Check sheet for the modelled part. Datum: model origin and axes. Units: mm. Face numbers are marked on the shaded views. Give positions to 0.01 mm unless a question says otherwise; leave off trailing zeros. Order: outer loops, then holes, each group sorted by start corner. A loop starts at its lowest first (then second) coordinate and runs counter-clockwise, first axis right, second up.
Item 1: Sectioned sample at A-A on x = 76.2. Record the boundary of the cut face in (y, z) (1 decimal).
Item 2: Release check for a two-part mould opening along Y. For the marked faces 1, 2, 3 and 4 record: released by +Y, released by -Y, zero draft, split by the parting line, or undercut.
Item 3: Sectioned sample at C-C on y = 6.5. Count the separate pieces of the cut face and the enclosed holes in it, and give its area (3 significant figures).
Item 4: Gauge pin test, flat ends, axial feed: P1, Ø6.5, axis at x = 109.54, y = 7.94, coming from the +Z side; P2, Ø7.5, axis at x = 46.04, y = 7.94, coming from the -Z side. Record the tip position at first contact, or that the pin passes through.
Item 5: Sectioned sample at B-B on x = 63.5. Record the boundary of the cut face in (y, z) (3 decimals).
Item 6: Material ranges on line 1 along X through (y, z) = (4.5, 12.25) (3 decimals); line 2 along X through (y, z) = (10, 7) (3 decimals); line 3 along X through (y, z) = (8.5, 13) (3 decimals), recorded low to high.
from build123d import *

# Parameters (mm, degrees)
F0_W     = 117.475
F0_H     = 15.875
F1_DEPTH = 25.4
F2_R     = 3.96875
F2_R_2   = 3.175
F2_R_3   = 5.55625
F3_DEPTH = 25.401
F4_R     = 3.175
F4_R_2   = 2.38125
F5_DEPTH = 15.876
F6_SIZE  = 0.762


with BuildPart() as f1:
    # F0 (on Top) → F1 (new body)
    with BuildSketch(Plane.XY):
        with Locations((58.7375, 7.9375)):
            Rectangle(F0_W, F0_H)
    extrude(amount=F1_DEPTH)

    # F2 (on face) → F3 (cut, through all)
    with BuildSketch(Plane.XY.offset(25.4)):
        with Locations((7.9375, 7.9375)):
            Circle(F2_R)
        with Locations((46.0375, 7.9375)):
            Circle(F2_R_2)
        with Locations((63.5, 7.9375)):
            Circle(F2_R_3)
        with Locations((109.5375, 7.9375)):
            Circle(F2_R)
    extrude(amount=-F3_DEPTH, mode=Mode.SUBTRACT)

    # F4 (on face) → F5 (cut, through all)
    with BuildSketch(Plane.XZ):
        with Locations((76.2, 17.4625)):
            Circle(F4_R)
        with Locations((90.4875, 5.5626)):
            Circle(F4_R_2)
    extrude(amount=-F5_DEPTH, mode=Mode.SUBTRACT)

    # F6
    f6_edges = [f1.edges().sort_by_distance(p)[0] for p in [
        (73.025, 0, 17.4625),
        (88.10625, 0, 5.5626),
        (57.94375, 7.9375, 25.4),
        (42.8625, 7.9375, 25.4),
        (105.56875, 7.9375, 25.4),
        (58.7375, 0, 25.4),
        (58.7375, 0, 0),
        (117.475, 0, 12.7),
        (0, 0, 12.7),
        (0, 7.9375, 25.4),
        (0, 15.875, 12.7),
        (0, 7.9375, 0),
        (58.7375, 15.875, 0),
        (3.96875, 7.9375, 0),
        (42.8625, 7.9375, 0),
        (57.94375, 7.9375, 0),
        (58.7375, 15.875, 25.4),
        (73.025, 15.875, 17.4625),
        (88.10625, 15.875, 5.5626),
        (3.96875, 7.9375, 25.4),
        (117.475, 7.9375, 25.4),
        (117.475, 15.875, 12.7),
        (117.475, 7.9375, 0),
        (105.56875, 7.9375, 0),
    ]]
    chamfer(f6_edges, length=F6_SIZE)


solid = f1.part
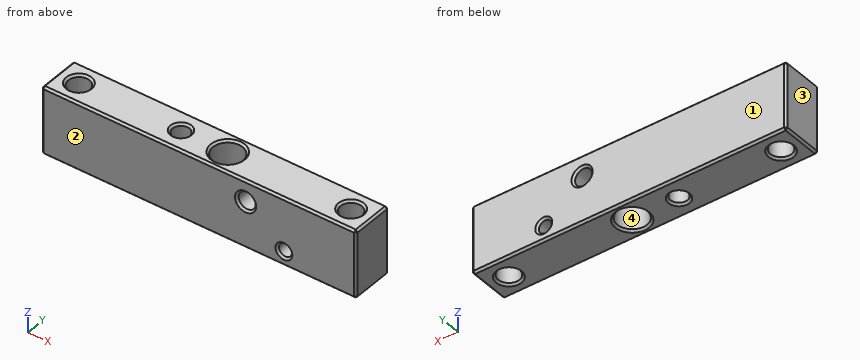
Report:
1. outline: (0, 0.8) - (0.8, 0) - (15.1, 0) - (15.9, 0.8) - (15.9, 13.5) - (15.1, 14.3) - (0.8, 14.3) - (0, 13.5) - close; (0, 21.4) - (0.8, 20.6) - (15.1, 20.6) - (15.9, 21.4) - (15.9, 24.6) - (15.1, 25.4) - (0.8, 25.4) - (0, 24.6) - close
2. face 1: released by +Y
2. face 2: released by -Y
2. face 3: zero draft
2. face 4: undercut
3. separate pieces: 5
3. enclosed holes: 2
3. area: 2,140 mm2
4. P1: passes through
4. P2: stops at z = 0.18
5. outline: (0, 0.762) - (0.762, 0) - (1.619, 0) - (2.381, 0.762) - (2.381, 24.638) - (1.619, 25.4) - (0.762, 25.4) - (0, 24.638) - close; (13.494, 0.762) - (14.256, 0) - (15.113, 0) - (15.875, 0.762) - (15.875, 24.638) - (15.113, 25.4) - (14.256, 25.4) - (13.494, 24.638) - close
6. line 1: x = 0 to 5.954, 9.921 to 59.135, 67.865 to 107.554, 111.521 to 117.475
6. line 2: x = 0 to 4.547, 11.328 to 43.624, 48.451 to 58.341, 68.659 to 88.589, 92.386 to 106.147, 112.928 to 117.475
6. line 3: x = 0 to 4.009, 11.866 to 42.913, 49.162 to 57.972, 69.028 to 105.609, 113.466 to 117.475
